Autodesk Inventor part; units mm, degrees
ref_plane "YZ Plane" through (0, 0, 0) normal (1, 0, 0) x (0, 1, 0)
ref_plane "XZ Plane" through (0, 0, 0) normal (0, 1, 0) x (-1, 0, 0)
ref_plane "XY Plane" through (0, 0, 0) normal (0, 0, 1) x (1, 0, 0)
sketch "スケッチ1" plane through (0, 0, 0) normal (0, 1, 0) x (-1, 0, 0)
  circle A0 centre (0, 0) radius 8
  dimension "d0" = 16
extrude "押し出し1" add sketch "スケッチ1" along normal blind 7
sketch "スケッチ2" plane through (0, 7, 0) normal (0, 1, 0) x (1, 0, 0)
  circle A0 centre (0, 0) radius 11.5
  dimension "d3" = 23
extrude "押し出し2" add sketch "スケッチ2" along normal blind 6
sketch "スケッチ3" plane through (0, 13, 0) normal (0, 1, 0) x (1, 0, 0)
  circle A0 centre (0, 0) radius 15
  dimension "d6" = 30
extrude "押し出し3" add sketch "スケッチ3" along normal blind 14
fillet "フィレット1" radius 5 1 edges at (-15, 27, 0)
sketch "スケッチ4" plane through (0, 0, 0) normal (0, -1, 0) x (1, 0, 0)
  line L0 (8, 9) -> (-8, 9)
  line L1 (-8, 9) -> (-8, -9)
  line L2 (-8, -9) -> (8, -9)
  line L3 (8, -9) -> (8, 9)
  circle A0 centre (0, 0) radius 10
  line L4 (8, 9) -> (-8, -9) construction
  line L5 (-8, 9) -> (8, -9) construction
  dimension "d10" = 16
  dimension "d11" = 18
extrude "押し出し4" add sketch "スケッチ4" along normal blind 10 contours L3 A0 L0 | A0 L3 L2 L1 L0 | A0 L1 L0 | L3 L2 A0 | A0 L2 L1
sketch "スケッチ5" plane through (0, -10, 0) normal (0, -1, 0) x (1, 0, 0)
  line L0 (-6, 8) -> (-6.2, 8)
  line L1 (-6.2, 8) -> (-6.2, 5)
  line L2 (-6.2, 5) -> (-6, 5)
  line L3 (-6, 5) -> (-6, 8)
  line L4 (6.2, 8) -> (6, 8)
  line L5 (6, 8) -> (6, 5)
  line L6 (6, 5) -> (6.2, 5)
  line L7 (6.2, 5) -> (6.2, 8)
  line L8 (0, -21) -> (0, 21)
  line L9 (8, 9) -> (-8, 9)
  point P0 (0, 0)
  point P1 (6.1, 8)
  dimension "d14" = 0.2
  dimension "d15" = 3
  dimension "d16" = 6
  dimension "d17" = 1
extrude "押し出し5" add sketch "スケッチ5" along normal blind 6
properties part number "emergency_button"
The listing builds one solid part. Answer for the finished solid, in the listing's coordinates (mm). A direction names the side the tool comes from. Round coordinates to 2 decimals unless told otherwise and drop trailing zeros. Loops run counter-clockwise (first coordinate to the right, second up) from the corner with the lowest first, then second, coordinate; pieces in that order, holes last. Notation, with made-up numbers: (39, 7.5) - (72, 7.5) arc R25 cw to (72, 25.5) - close; hole circle Ø9 at (61.5, 41.5). An arc over 180 degrees is marked (long way). Use one line per item in the form item = value. Start each with the question number.
1. A tool of negligible diameter and unlimited length cuts with its end or side. For faces 1 (the face through (-8, 7, 2)), 2 (the face through (6.2, -13, 6)), 3 (the face through (-8, -5, 0)), from which of +Z, -Z, +X, -X, +Y, -Y can it reach the whole face along a straight path? Write none if from no direction.
2. The part is cut by section C-C on y = -0.5. Determine the outline of the cut face in (x, z).
3. Given pin 1 Ø5 at (x, y) = (-2.5, -5.5) entering from +Z; pin 2 Ø2.5 at (y, z) = (-14, 7) entering from -X; pin 3 Ø1.5 at (x, y) = (4, 4.5) entering from +Z; pin 4 Ø5 at (x, z) = (2, 10.5) entering from +Y, each flat-ended and moving along its own axis, determine where each tip first touches the part or whether it passes through.
4. The part is cut by section A-A on y = -12. Determine the outline of the cut face in (x, z), then the cut area to 3 significant figures.
5. For a pull along Y with two mould halves and no side action, classify faces 4 (the face through (0, 27, 0)), 5 (the face through (1.73, 3.45, 7.81)), 6 (the face through (-6, -13, 6)) as pulls with the +Y half, pulls with the -Y half, needs draft (parallel to the pull), parting line crosses it, or undercut.
6. The part is cut by section D-D on y = 19. Determine the outline of the cut face in (x, z).
7. Consider line 1 (Y direction, x = 3.5, z = -6.75); line 2 (Y direction, x = 6.25, z = 8); line 3 (X direction, y = 15, z = -6). Determine where each line is inside the solid, lowest interval first. Write a range as [from, to].
8. The part is cut by section B-B on x = 0. Determine the outline of the cut face in (y, z), then the cut area to 3 significant figures.
Geometry check:
q1.face_1 = none
q1.face_2 = +Z, -Z, +X, -Y
q1.face_3 = +Z, -Z, -X, -Y
q2.outline = (-8, -9) - (8, -9) - (8, 9) - (-8, 9) - close
q3.pin_1 = 9
q3.pin_2 = -6.2
q3.pin_3 = 7.31
q3.pin_4 = 27
q4.outline = (-6.2, 5) - (-6, 5) - (-6, 8) - (-6.2, 8) - close; (6, 5) - (6.2, 5) - (6.2, 8) - (6, 8) - close
q4.area = 1.20 mm^2
q5.face_4 = pulls with the +Y half
q5.face_5 = undercut
q5.face_6 = needs draft
q6.outline = circle Ø30 at (0, 0)
q7.line_1 = [-10, 27]
q7.line_2 = [-10, 0], [7, 27]
q7.line_3 = [-13.75, 13.75]
q8.outline = (-10, -9) - (0, -9) - (0, -8) - (7, -8) - (7, -11.5) - (13, -11.5) - (13, -15) - (22, -15) arc R5 ccw to (27, -10) - (27, 10) arc R5 ccw to (22, 15) - (13, 15) - (13, 11.5) - (7, 11.5) - (7, 8) - (0, 8) - (0, 9) - (-10, 9) - close
q8.area = 839 mm^2
